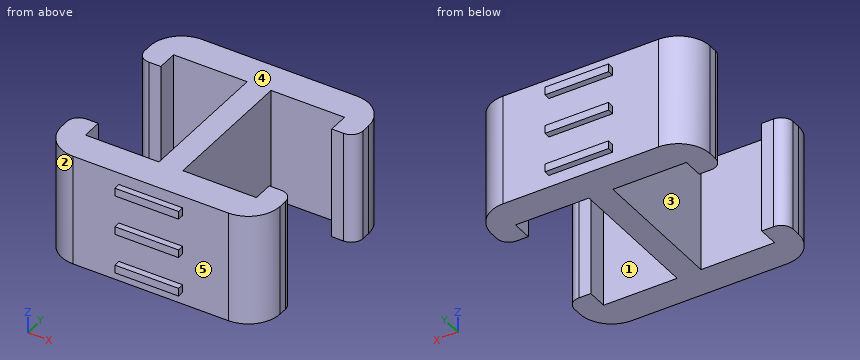
```python
from build123d import *

# Parameters (mm, degrees)
F0_W     = 1.5
F0_H     = 8.75
F1_DEPTH = 7
F2_R     = 0.75
F3_R     = 2
F4_W     = 4
F4_H     = 0.5
F5_DEPTH = 0.4
F6_W     = 4
F6_H     = 0.5
F7_DEPTH = 0.4


# Not quite as in the source:
# - a feature names something its author has since deleted; it is built from what else it names


with BuildPart() as f1:
    # F0 (on Top) → F1 (new body)
    with BuildSketch(Plane.XY):
        Polygon((5.375, -4.375), (0.75, -4.375), (-0.75, -4.375), (-5.375, -4.375), (-5.375, -6.375), (5.375, -6.375), align=None)
        Rectangle(F0_W, F0_H)
        Polygon((-0.75, 4.375), (0.75, 4.375), (5.375, 4.375), (5.375, 6.375), (-5.375, 6.375), (-5.375, 4.375), align=None)
        Polygon((5.375, -3.1), (5.375, -4.375), (5.375, -6.375), (6.875, -6.375), (6.875, -3.1), align=None)
        Polygon((-5.375, -6.375), (-5.375, -4.375), (-5.375, -3.1), (-6.875, -3.1), (-6.875, -6.375), align=None)
        Polygon((5.375, 6.375), (5.375, 4.375), (5.375, 3.1), (6.875, 3.1), (6.875, 6.375), align=None)
        Polygon((-5.375, 3.1), (-5.375, 4.375), (-5.375, 6.375), (-6.875, 6.375), (-6.875, 3.1), align=None)
    extrude(amount=F1_DEPTH)

    # F2
    f2_edges = [f1.edges().sort_by_distance(p)[0] for p in [
        (-6.875, 3.1, 3.5),
        (6.875, 3.1, 3.5),
        (6.875, -3.1, 3.5),
        (-6.875, -3.1, 3.5),
    ]]
    fillet(f2_edges, radius=F2_R)

    # F3
    f3_edges = [f1.edges().sort_by_distance(p)[0] for p in [
        (-6.875, -6.375, 3.5),
        (6.875, -6.375, 3.5),
        (6.875, 6.375, 3.5),
        (-6.875, 6.375, 3.5),
    ]]
    fillet(f3_edges, radius=F3_R)

    # F4 (on face) → F5 (join)
    with BuildSketch(Plane(origin=(0, 6.375, 0), x_dir=(-1, 0, 0), z_dir=(0, 1, 0))):
        with Locations((0, 1)):
            Rectangle(F4_W, F4_H)
        with Locations((0, 3.5)):
            Rectangle(F4_W, F4_H)
        with Locations((0, 6)):
            Rectangle(F4_W, F4_H)
    extrude(amount=F5_DEPTH)

    # F6 (on face) → F7 (join)
    with BuildSketch(Plane.XZ.offset(6.375)):
        with Locations((0, 3.5)):
            Rectangle(F6_W, F6_H)
        with Locations((0, 6)):
            Rectangle(F6_W, F6_H)
        with Locations((0, 1)):
            Rectangle(F6_W, F6_H)
    extrude(amount=F7_DEPTH)


solid = f1.part
```
The listing builds one solid part. Answer for the finished solid, in the listing's coordinates (mm). Face numbers are marked on the shaded views. A direction names the side the tool comes from. Round coordinates to 2 decimals unless told otherwise and drop trailing zeros. Loops run counter-clockwise (first coordinate to the right, second up) from the corner with the lowest first, then second, coordinate; pieces in that order, holes last.
1) A cutting plane is placed at C-C on x = 4.25. Determine the outline of the cut face in (y, z) (3 decimals).
Outcome:
outline: (-6.375, 0) - (-4.375, 0) - (-4.375, 7) - (-6.375, 7) - close; (4.375, 0) - (6.375, 0) - (6.375, 7) - (4.375, 7) - close
2) Given P1, Ø2, axis at x = 4.5, z = 3, coming from the +Y side (3 decimals); P2, Ø4, axis at x = -3.5, z = 1, coming from the +Y side (3 decimals), each flat-ended and moving along its own axis, determine where each tip first touches the part or whether it passes through.
Outcome:
P1: stops at y = 6.375
P2: stops at y = 6.775
3) A cutting plane is placed at B-B on z = 3. Determine the outline of the cut face in (x, y) (3 decimals), plus the area to 3 significant figures.
Outcome:
outline: (-6.875, -4.375) arc R2 ccw to (-4.875, -6.375) - (4.875, -6.375) arc R2 ccw to (6.875, -4.375) - (6.875, -3.85) arc R0.75 ccw to (6.125, -3.1) - (5.375, -3.1) - (5.375, -4.375) - (0.75, -4.375) - (0.75, 4.375) - (5.375, 4.375) - (5.375, 3.1) - (6.125, 3.1) arc R0.75 ccw to (6.875, 3.85) - (6.875, 4.375) arc R2 ccw to (4.875, 6.375) - (-4.875, 6.375) arc R2 ccw to (-6.875, 4.375) - (-6.875, 3.85) arc R0.75 ccw to (-6.125, 3.1) - (-5.375, 3.1) - (-5.375, 4.375) - (-0.75, 4.375) - (-0.75, -4.375) - (-5.375, -4.375) - (-5.375, -3.1) - (-6.125, -3.1) arc R0.75 ccw to (-6.875, -3.85) - close
area: 71.9 mm2
4) For a pull along Z with two mould halves and no side action, classify the marked faces 3, 4 and 5 as released by +Z, released by -Z, zero draft, split by the parting line, or undercut.
Outcome:
face 3: zero draft
face 4: released by +Z
face 5: undercut
5) A cutting plane is placed at D-D on x = 0.5. Determine the outline of the cut face in (y, z) (3 decimals).
Outcome:
outline: (-6.775, 0.75) - (-6.375, 0.75) - (-6.375, 0) - (6.375, 0) - (6.375, 0.75) - (6.775, 0.75) - (6.775, 1.25) - (6.375, 1.25) - (6.375, 3.25) - (6.775, 3.25) - (6.775, 3.75) - (6.375, 3.75) - (6.375, 5.75) - (6.775, 5.75) - (6.775, 6.25) - (6.375, 6.25) - (6.375, 7) - (-6.375, 7) - (-6.375, 6.25) - (-6.775, 6.25) - (-6.775, 5.75) - (-6.375, 5.75) - (-6.375, 3.75) - (-6.775, 3.75) - (-6.775, 3.25) - (-6.375, 3.25) - (-6.375, 1.25) - (-6.775, 1.25) - close
6) For the marked faces 1 and 2, determine the directions among +Z, -Z, +X, -X, +Y, -Y from which every point of the face is accessible in a straight line to the end or side of a thin tool.
Outcome:
face 1: +Z, -Z
face 2: +Z, -Z, -X, -Y
7) Consider line 1 (Y direction, x = -4, z = 2.5) (3 decimals); line 2 (X direction, y = 0.5, z = 5); line 3 (Y direction, x = 0.25, z = 4) (3 decimals). Determine where each line is inside the solid, lowest interval first.
Outcome:
line 1: y = -6.375 to -4.375, 4.375 to 6.375
line 2: x = -0.75 to 0.75
line 3: y = -6.375 to 6.375
